Read the model definition and answer for the solid it produces. Units are mm, in the model's axes. Give positions to 0.01 mm unless a question says otherwise; leave off trailing zeros. Order: outer loops, then holes, each group sorted by start corner. A loop starts at its lowest first (then second) coordinate and runs counter-clockwise, first axis right, second up. Notation, with made-up numbers: (-22.75, 1.5) - (24.25, 1.5) arc R12 ccw to (24.25, 7.5) - close; hole circle Ø7 at (29, 67.5). An arc over 180 degrees is marked (long way). Write item = value, one per line.
```python
from build123d import *

# Parameters (mm, degrees)
SKETCH1_W           = 123
SKETCH1_H           = 50
BOSS_EXTRUDE1_DEPTH = 2.4
SKETCH2_W           = 50
SKETCH2_H           = 43
SKETCH2_W_2         = 44
SKETCH2_H_2         = 18
BOSS_EXTRUDE2_DEPTH = 5
SKETCH3_W           = 24.5
SKETCH3_H           = 50.5
SKETCH3_W_2         = 18.5
SKETCH3_H_2         = 44.5
BOSS_EXTRUDE3_DEPTH = 5
SKETCH4_W           = 11.5
SKETCH4_H           = 3
CUT_EXTRUDE2_DEPTH  = 3
SKETCH5_W           = 30
SKETCH5_H           = 33
SKETCH5_W_2         = 24
SKETCH5_H_2         = 27
BOSS_EXTRUDE5_DEPTH = 5
SKETCH6_W           = 36.9
SKETCH6_H           = 11.8
SKETCH6_W_2         = 7
SKETCH6_H_2         = 7
BOSS_EXTRUDE6_DEPTH = 8
SKETCH7_W           = 5.123641681
SKETCH7_H           = 1
CUT_EXTRUDE3_DEPTH  = 5
SKETCH8_W           = 3
SKETCH8_H           = 5.294429738
SKETCH8_H_2         = 5.550611822
SKETCH8_H_3         = 2.134850701
SKETCH8_H_4         = 2.647214869
SKETCH8_H_5         = 2.348335771
SKETCH8_H_6         = 2.903396953
SKETCH8_H_7         = 2.988790981
SKETCH8_H_8         = 6.233764046
SKETCH8_H_9         = 2.049456673
SKETCH8_H_10        = 2.1348507
SKETCH8_H_11        = 2.818002924
SKETCH8_H_12        = 2.476426813
SKETCH8_H_13        = 2.689911883
SKETCH8_H_14        = 2.775305911
SKETCH8_H_15        = 3.693291713
SKETCH8_W_2         = 8.561478369
SKETCH8_H_16        = 3
CUT_EXTRUDE4_DEPTH  = 5
SKETCH9_W           = 3.123120747
SKETCH9_H           = 2.4
SKETCH9_W_2         = 4.09656098
SKETCH9_W_3         = 3.163680757
SKETCH9_W_4         = 3.690960883
CUT_EXTRUDE5_DEPTH  = 8
SKETCH10_W          = 3
SKETCH10_H          = 3
SKETCH10_H_2        = 3.330367093
SKETCH10_H_3        = 4
CUT_EXTRUDE6_DEPTH  = 5


with BuildPart() as part:
    # Sketch1 → Boss-Extrude1 (new body)
    with BuildSketch(Plane(origin=(0, 0, 0), x_dir=(1, 0, 0), z_dir=(0, 1, 0))):
        with Locations((61.5, -25)):
            Rectangle(SKETCH1_W, SKETCH1_H)
    extrude(amount=BOSS_EXTRUDE1_DEPTH)

    # Sketch2 → Boss-Extrude2 (add)
    with BuildSketch(Plane(origin=(0, 2.4, 0), x_dir=(1, 0, 0), z_dir=(0, 1, 0))):
        with Locations((27, -25)):
            Rectangle(SKETCH2_W, SKETCH2_H)
        with Locations((27, -15.5)):
            Rectangle(SKETCH2_W_2, SKETCH2_H_2, mode=Mode.SUBTRACT)
        with Locations((27, -34.5)):
            Rectangle(SKETCH2_W_2, SKETCH2_H_2, mode=Mode.SUBTRACT)
    extrude(amount=BOSS_EXTRUDE2_DEPTH)

    # Sketch3 → Boss-Extrude3 (add)
    with BuildSketch(Plane(origin=(0, 2.4, 0), x_dir=(1, 0, 0), z_dir=(0, 1, 0))):
        with Locations((71.25, -25)):
            Rectangle(SKETCH3_W, SKETCH3_H)
        with Locations((71.25, -25)):
            Rectangle(SKETCH3_W_2, SKETCH3_H_2, mode=Mode.SUBTRACT)
    extrude(amount=BOSS_EXTRUDE3_DEPTH)

    # Sketch4 → Cut-Extrude2 (cut)
    with BuildSketch(Plane(origin=(0, 7.4, 0), x_dir=(1, 0, 0), z_dir=(0, 1, 0))):
        with Locations((71.25, -1.25)):
            Rectangle(SKETCH4_W, SKETCH4_H)
    extrude(amount=-CUT_EXTRUDE2_DEPTH, mode=Mode.SUBTRACT)

    # Sketch5 → Boss-Extrude5 (add)
    with BuildSketch(Plane(origin=(0, 2.4, 0), x_dir=(1, 0, 0), z_dir=(0, 1, 0))):
        with Locations((105.5, -31.5)):
            Rectangle(SKETCH5_W, SKETCH5_H)
        with Locations((105.5, -31.5)):
            Rectangle(SKETCH5_W_2, SKETCH5_H_2, mode=Mode.SUBTRACT)
    extrude(amount=BOSS_EXTRUDE5_DEPTH)

    # Sketch6 → Boss-Extrude6 (add)
    with BuildSketch(Plane(origin=(0, 2.4, 0), x_dir=(1, 0, 0), z_dir=(0, 1, 0))):
        with Locations((104.55, -6.5)):
            Rectangle(SKETCH6_W, SKETCH6_H)
        with Locations((92, -6.5)):
            Rectangle(SKETCH6_W_2, SKETCH6_H_2, mode=Mode.SUBTRACT)
        with Locations((100.5, -6.5)):
            Rectangle(SKETCH6_W_2, SKETCH6_H_2, mode=Mode.SUBTRACT)
        with Locations((109, -6.5)):
            Rectangle(SKETCH6_W_2, SKETCH6_H_2, mode=Mode.SUBTRACT)
        with Locations((117.5, -6.5)):
            Rectangle(SKETCH6_W_2, SKETCH6_H_2, mode=Mode.SUBTRACT)
    extrude(amount=BOSS_EXTRUDE6_DEPTH)

    # Sketch7 → Cut-Extrude3 (cut)
    with BuildSketch(Plane(origin=(0, 7.4, 0), x_dir=(1, 0, 0), z_dir=(0, 1, 0))):
        with Locations((44.079618283, -25)):
            Rectangle(SKETCH7_W, SKETCH7_H)
    extrude(amount=-CUT_EXTRUDE3_DEPTH, mode=Mode.SUBTRACT)

    # Sketch8 → Cut-Extrude4 (cut)
    with BuildSketch(Plane(origin=(0, 7.4, 0), x_dir=(1, 0, 0), z_dir=(0, 1, 0))):
        with Locations((50.5, -15.563959903)):
            Rectangle(SKETCH8_W, SKETCH8_H)
        with Locations((50.5, -35.418071419)):
            Rectangle(SKETCH8_W, SKETCH8_H_2)
        with Locations((60.5, -10.056045096)):
            Rectangle(SKETCH8_W, SKETCH8_H_3)
        with Locations((60.5, -16.887567338)):
            Rectangle(SKETCH8_W, SKETCH8_H_4)
        with Locations((60.5, -23.825832115)):
            Rectangle(SKETCH8_W, SKETCH8_H_5)
        with Locations((60.5, -31.191067032)):
            Rectangle(SKETCH8_W, SKETCH8_H_6)
        with Locations((60.5, -38.236074344)):
            Rectangle(SKETCH8_W, SKETCH8_H_7)
        with Locations((82, -10.397621207)):
            Rectangle(SKETCH8_W, SKETCH8_H_8)
        with Locations((82, -20.175237417)):
            Rectangle(SKETCH8_W, SKETCH8_H_9)
        with Locations((82, -25.42697014)):
            Rectangle(SKETCH8_W, SKETCH8_H_10)
        with Locations((82, -31.191067032)):
            Rectangle(SKETCH8_W, SKETCH8_H_6)
        with Locations((82, -37.55292212)):
            Rectangle(SKETCH8_W, SKETCH8_H_11)
        with Locations((82, -43.188927969)):
            Rectangle(SKETCH8_W, SKETCH8_H_12)
        with Locations((92, -26.771926082)):
            Rectangle(SKETCH8_W, SKETCH8_H_13)
        with Locations((92, -32.685462523)):
            Rectangle(SKETCH8_W, SKETCH8_H_7)
        with Locations((92, -38.940575076)):
            Rectangle(SKETCH8_W, SKETCH8_H_14)
        with Locations((119, -40.787220932)):
            Rectangle(SKETCH8_W, SKETCH8_H_15)
        with Locations((119, -24.039317184)):
            Rectangle(SKETCH8_W, SKETCH8_H_14)
        with Locations((101.219260816, -16.5)):
            Rectangle(SKETCH8_W_2, SKETCH8_H_16)
    extrude(amount=-CUT_EXTRUDE4_DEPTH, mode=Mode.SUBTRACT)

    # Sketch9 → Cut-Extrude5 (cut)
    with BuildSketch(Plane(origin=(0, 10.4, 0), x_dir=(1, 0, 0), z_dir=(0, 1, 0))):
        with Locations((92.086007163, -11.2)):
            Rectangle(SKETCH9_W, SKETCH9_H)
        with Locations((100.441369161, -11.2)):
            Rectangle(SKETCH9_W_2, SKETCH9_H)
        with Locations((108.938691194, -11.2)):
            Rectangle(SKETCH9_W_3, SKETCH9_H)
        with Locations((117.476573236, -11.2)):
            Rectangle(SKETCH9_W_4, SKETCH9_H)
    extrude(amount=-CUT_EXTRUDE5_DEPTH, mode=Mode.SUBTRACT)

    # Sketch10 → Cut-Extrude6 (cut)
    with BuildSketch(Plane(origin=(0, 7.4, 0), x_dir=(1, 0, 0), z_dir=(0, 1, 0))):
        with Locations((3.5, -11)):
            Rectangle(SKETCH10_W, SKETCH10_H)
        with Locations((3.5, -17.485325534)):
            Rectangle(SKETCH10_W, SKETCH10_H_2)
        with Locations((3.5, -30.63600585)):
            Rectangle(SKETCH10_W, SKETCH10_H_2)
        with Locations((3.5, -38.5)):
            Rectangle(SKETCH10_W, SKETCH10_H_3)
    extrude(amount=-CUT_EXTRUDE6_DEPTH, mode=Mode.SUBTRACT)


solid = part.part
```
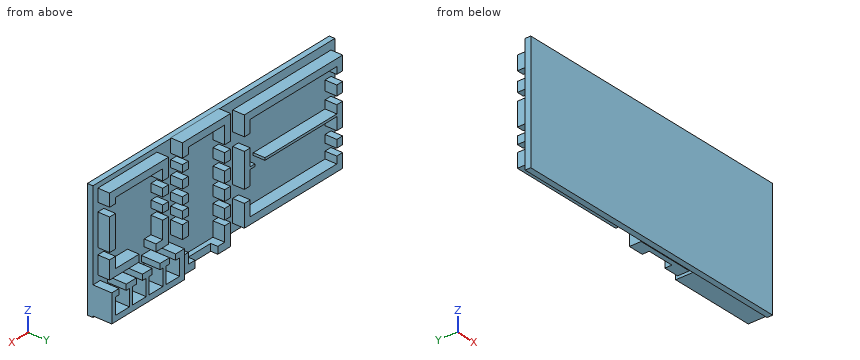
1. Flat-ended cylindrical pins translate along their axes: pin 1 (0.9 mm diameter, centred on x = 4, y = 4, fed in from -Z); pin 2 (2 mm diameter, centred on y = 4.5, z = 13, fed in from -X); pin 3 (3.5 mm diameter, centred on x = 102, y = 5.5, fed in from +Z). Find the tip coordinate at first contact, or state that the pin passes through.
Recorded:
pin_1 = 3.5
pin_2 = 2
pin_3 = 48
2. Section D-D (x = 57) is taken. Determine the outline of the cut face in (y, z).
Recorded:
outline = (0, 0) - (2.4, 0) - (2.4, 50) - (0, 50) - close
3. Section A-A (x = 14) is taken. Determine the outline of the cut face in (y, z).
Recorded:
outline = (0, 0) - (2.4, 0) - (2.4, 3.5) - (7.4, 3.5) - (7.4, 6.5) - (2.4, 6.5) - (2.4, 24.5) - (7.4, 24.5) - (7.4, 25.5) - (2.4, 25.5) - (2.4, 43.5) - (7.4, 43.5) - (7.4, 46.5) - (2.4, 46.5) - (2.4, 50) - (0, 50) - close
4. Straight lines are drawn through the part: L1, parallel to Z at x = 48, y = 6; L2, parallel to X at y = 4.25, z = 46; L3, parallel to X at y = 2.75, z = 31. For each, find the intervals that lie inside material, in ascending order. Write a range as [from, to].
Recorded:
L1 = [3.5, 6.5], [24.5, 25.5], [43.5, 46.5]
L2 = [2, 52], [59, 62], [80.5, 83.5], [90.5, 120.5]
L3 = [49, 52], [90.5, 93.5], [117.5, 120.5]
5. Section B-B (y = 6.25) is taken. Count the separate pieces of the cut face and the enclosed holes in it, and give its area (3 significant figures).
Recorded:
separate_pieces = 25
enclosed_holes = 0
area = 1,250 mm^2
6. Section C-C (x = 44) is taken. Determine the outline of the cut face in (y, z).
Recorded:
outline = (0, 0) - (2.4, 0) - (2.4, 3.5) - (7.4, 3.5) - (7.4, 6.5) - (2.4, 6.5) - (2.4, 43.5) - (7.4, 43.5) - (7.4, 46.5) - (2.4, 46.5) - (2.4, 50) - (0, 50) - close
